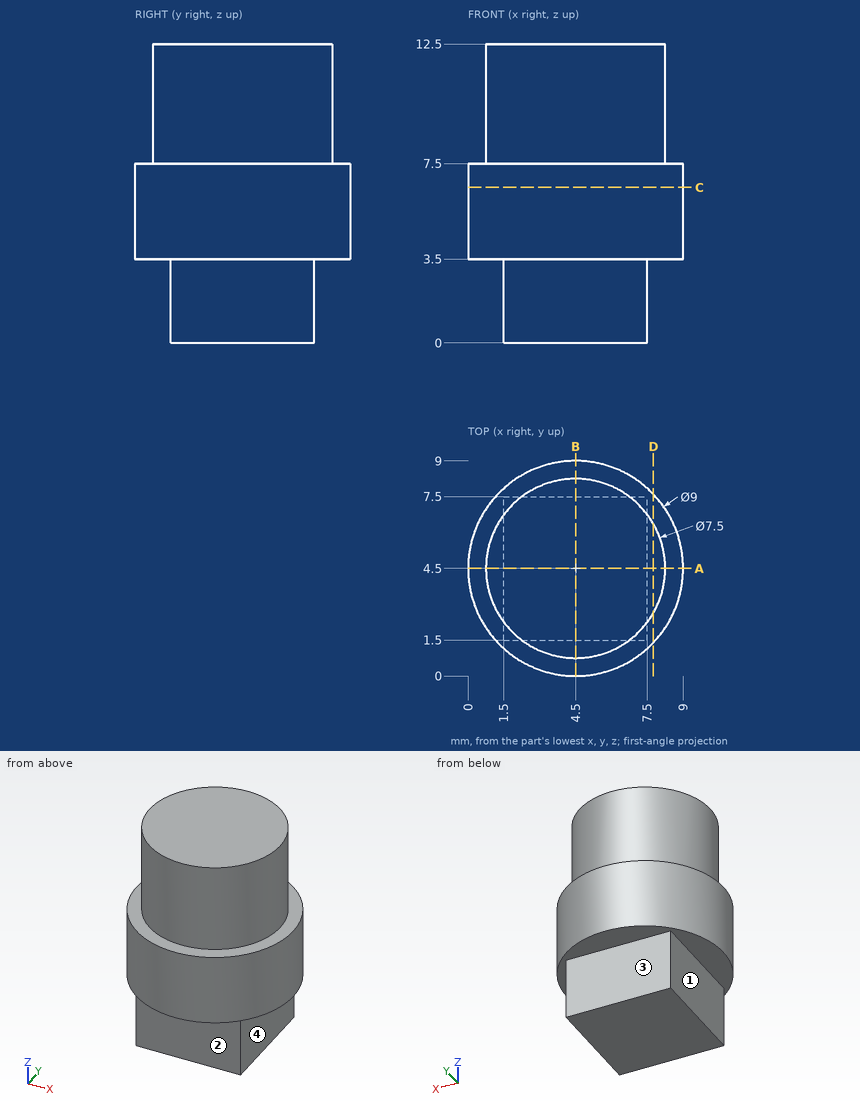
Part print with two shaded views. Sizes in mm from the minimum x, y, z corner. A direction names the side the tool comes from. Round coordinates to 2 decimals unless told otherwise and drop trailing zeros. Write each loop counter-clockwise with the first axis right and the second up, starting at its lowest first coordinate (ties: lowest second). Pieces come first, ordered by that corner, then holes. Notation, with made-up numbers: M 12.25,1 L 50.25,1 A13 ccw 50.25,5 Z; hole C -16,3 d9. An arc over 180 degrees is marked long. Answer as CSV lines item,"result". Start each with the question number.
1) Which spindle directions (+Z, -Z, +X, -X, +Y, -Y) get a long thin tool onto all of the face, cutting with end or side? Do the marked faces 1, 2, 3 and 4. Say none if no direction does.
2) Drill centre lines: L1, parallel to Z at x = 8, y = 4; L2, parallel to Y at x = 6, z = 2.75. Where is each one in solid material? Low to high.
3) Drop flat-ended pins along their axis: pin 1 (1.5 mm diameter, centred on x = 3.5, z = 4, fed in from -Y); pin 2 (1.5 mm diameter, centred on y = 3, z = 6.5, fed in from -X); pin 3 (1.5 mm diameter, centred on y = 5.5, z = 6.5, fed in from -X). Give the stop position or say it passes through.
4) Band-saw the part on D-D (x = 7.75). List the corners of the cut face in (y, z).
5) Band-saw the part on C-C (z = 6.5). List the corners of the cut face in (x, y).
6) Band-saw the part on A-A (y = 4.5). List the corners of the cut face in (x, z).
Worked out:
1,face 1,"-Z, -X, +Y, -Y"
1,face 2,"-Z, +X, -X, -Y"
1,face 3,"-Z, +X, -X, +Y"
1,face 4,"-Z, +X, +Y, -Y"
2,L1,"3.5 to 12.5"
2,L2,"1.5 to 7.5"
3,pin 1,"y = 0.01"
3,pin 2,"x = 0.06"
3,pin 3,"x = 0.01"
4,outline,"M 1.39,3.5 L 7.61,3.5 L 7.61,7.5 L 6.37,7.5 L 6.37,12.5 L 2.63,12.5 L 2.63,7.5 L 1.39,7.5 Z"
5,outline,"C 4.5,4.5 d9"
6,outline,"M 0,3.5 L 1.5,3.5 L 1.5,0 L 7.5,0 L 7.5,3.5 L 9,3.5 L 9,7.5 L 8.25,7.5 L 8.25,12.5 L 0.75,12.5 L 0.75,7.5 L 0,7.5 Z"
